Input: part model. Units: mm. Frame: model coordinates. A direction names the side the tool comes from. Give positions to 0.01 mm unless a question says otherwise; leave off trailing zeros. Loops run counter-clockwise (first coordinate to the right, second up) from the corner with the lowest first, then second, coordinate; pieces in that order, holes last. Notation, with made-up numbers: (3.25, 58.5) - (60.25, 58.5) arc R11 ccw to (60.25, 76.5) - close; hole circle Ø2 at (-20.75, 9.5). An arc over 180 degrees is marked (long way). Answer as a JSON object with one key per item and string values. Group by question number.
(1) Section query C-C (z = 16). Return loops of the section in (x, y), plus the area to 3 significant figures.
(2) Material intervals for L1, parallel to Y at x = 0, z = 5.5; L2, parallel to Y at x = -11.5, z = 39; L3, parallel to Z at x = 0, y = -6, sorted ascending.
(3) Section query B-B (y = 0). Return loops of the section in (x, z), plus the area to 3 significant figures.
(4) Section query D-D (y = 7). Return loops of the section in (x, z).
(5) Pin query (flat end, axial travel): P1, Ø1.2, axis at x = 11.5, y = -1, coming from the +Z side; P2, Ø1, axis at x = -5.5, z = 21.5, coming from the +Y side; P3, Ø12, axis at x = 1, z = 38.5, coming from the -Y side. Return the tip coordinate at first contact, or that it passes through.
(6) Section query A-A (x = 0). Return loops of the section in (y, z), plus the area to 3 significant figures.
(7) Mould query, pull axis X, two halves, no side actions, for faces 1 (the cylindrical face through (0, -14, 12)), 2 (the flat face through (14, -5.5, 11)), 3 (the cylindrical face through (-0.91, 6.34, 23.06)), 4 (the cylindrical face through (-9.21, -0.049, 23.985)). Classes: +X half, -X half, draft (parallel to the pull), parting line (faces both ways), or undercut.
(8) Access query for faces 5 (the cylindrical face through (0, 14, 12)), 6 (the flat face through (14, 5.5, 11)), 7 (the cylindrical face through (4.707, -9.049, 9.86)). Directions: +Z, -Z, +X, -X, +Y, -Y. A direction counts if a zero-diameter tool reaches every point of the face in a straight line with its end or side. Return the directions, or none.
```python
from build123d import *

# Parameters (mm, degrees)
CYLINDER002_R          = 11
CYLINDER002_DEPTH      = 7
CYLINDER002_ROLL_ANGLE = -90
BOX_W                  = 30
BOX_H                  = 7
BOX_DEPTH              = 15
BOX001_W               = 10
BOX001_H               = 7
BOX001_DEPTH           = 30
CYLINDER005_R          = 10.2
CYLINDER005_DEPTH      = 20
CYLINDER004_R          = 7
CYLINDER004_DEPTH      = 30
CYLINDER004_ROLL_ANGLE = -90
CYLINDER001_R          = 15
CYLINDER001_DEPTH      = 15
CYLINDER001_ROLL_ANGLE = -90
BOX002_W               = 30
BOX002_H               = 11
BOX002_DEPTH           = 30
CYLINDER_R             = 14
CYLINDER_DEPTH         = 24


with BuildPart() as cylinder002:
    # Cylinder002 → Cylinder002 (new body)
    with BuildSketch(Plane.XY):
        Circle(CYLINDER002_R)
    extrude(amount=CYLINDER002_DEPTH)


with BuildPart() as cylinder002_1:
    # Cylinder002 roll: moved
    add(cylinder002.part.rotate(Axis((0, 0, 0), (1, 0, 0)), CYLINDER002_ROLL_ANGLE))


with BuildPart() as cylinder002_2:
    # Cylinder002 placement: moved
    add(cylinder002_1.part.moved(Location((0, -3.5, 30))))


with BuildPart() as cube:
    # Box → Box (new body)
    with BuildSketch(Plane(origin=(-15, -3.5, 30), x_dir=(1, 0, 0), z_dir=(0, 0, 1))):
        with Locations((15, 3.5)):
            Rectangle(BOX_W, BOX_H)
    extrude(amount=BOX_DEPTH)


with BuildPart() as cube001:
    # Box001 → Box001 (new body)
    with BuildSketch(Plane(origin=(12.5, -3.5, 0), x_dir=(1, 0, 0), z_dir=(0, 0, 1))):
        with Locations((5, 3.5)):
            Rectangle(BOX001_W, BOX001_H)
    extrude(amount=BOX001_DEPTH)


with BuildPart() as cylinder005:
    # Cylinder005 → Cylinder005 (new body)
    with BuildSketch(Plane.XY):
        Circle(CYLINDER005_R)
    extrude(amount=CYLINDER005_DEPTH)


with BuildPart() as obj1:
    # Cylinder004 → Cylinder004 (new body)
    with BuildSketch(Plane.XY):
        Circle(CYLINDER004_R)
    extrude(amount=CYLINDER004_DEPTH)


with BuildPart() as obj1_1:
    # Cylinder004 roll: moved
    add(obj1.part.rotate(Axis((0, 0, 0), (1, 0, 0)), CYLINDER004_ROLL_ANGLE))


with BuildPart() as obj1_2:
    # Cylinder004 placement: moved
    add(obj1_1.part.moved(Location((0, -15, 30))))

    # Fusion001: union Cylinder002, Cube, Cube001, Cylinder005
    add(cylinder002_2.part)
    add(cube.part)
    add(cube001.part)
    add(cylinder005.part)


with BuildPart() as cylinder001:
    # Cylinder001 → Cylinder001 (new body)
    with BuildSketch(Plane.XY):
        Circle(CYLINDER001_R)
    extrude(amount=CYLINDER001_DEPTH)


with BuildPart() as cylinder001_1:
    # Cylinder001 roll: moved
    add(cylinder001.part.rotate(Axis((0, 0, 0), (1, 0, 0)), CYLINDER001_ROLL_ANGLE))


with BuildPart() as cylinder001_2:
    # Cylinder001 placement: moved
    add(cylinder001_1.part.moved(Location((0, -7.5, 30))))


with BuildPart() as cube002:
    # Box002 → Box002 (new body)
    with BuildSketch(Plane(origin=(-15, -5.5, 0), x_dir=(1, 0, 0), z_dir=(0, 0, 1))):
        with Locations((15, 5.5)):
            Rectangle(BOX002_W, BOX002_H)
    extrude(amount=BOX002_DEPTH)


with BuildPart() as cut:
    # Cylinder → Cylinder (new body)
    with BuildSketch(Plane.XY):
        Circle(CYLINDER_R)
    extrude(amount=CYLINDER_DEPTH)

    # Fusion: union Cylinder001, Cube002
    add(cylinder001_2.part)
    add(cube002.part)

    # Cut: cut obj1
    add(obj1_2.part, mode=Mode.SUBTRACT)


solid = cut.part
```
Recorded:
{
 "1": {"outline": "(-15, -5.5) - (-12.87, -5.5) arc R14 ccw to (12.87, -5.5) - (15, -5.5) - (15, -3.5) - (12.5, -3.5) - (12.5, 3.5) - (15, 3.5) - (15, 5.5) - (12.87, 5.5) arc R14 ccw to (-12.87, 5.5) - (-15, 5.5) - close; hole circle Ø20.4 at (0, 0)", "area": "302 mm^2"},
 "2": {"L1": "y = -14 to -10.2, 10.2 to 14", "L2": "y = -7.5 to -3.5, 3.5 to 7.5", "L3": "z = 20 to 23, 37 to 45"},
 "3": {"outline": "(-15, 0) - (-10.2, 0) - (-10.2, 20) - (-4.58, 20) arc R11 cw to (-11, 30) - (-15, 30) - close; (4.58, 20) - (10.2, 20) - (10.2, 0) - (12.5, 0) - (12.5, 30) - (11, 30) arc R11 cw to start", "area": "233 mm^2"},
 "4": {"outline": "(-12.12, 0) - (-7.42, 0) - (-7.42, 20) - (7.42, 20) - (7.42, 0) - (12.12, 0) - (12.12, 21.17) arc R15 ccw (long way) to (-12.12, 21.17) - close; hole circle Ø14 at (0, 30)"},
 "5": {"P1": "stops at z = 30", "P2": "stops at y = 13.08", "P3": "stops at y = -7.5"},
 "6": {"outline": "(-14, 0) - (-10.2, 0) - (-10.2, 20) - (-3.5, 20) - (-3.5, 23) - (-14, 23) - close; (-7.5, 37) - (-3.5, 37) - (-3.5, 45) - (-7.5, 45) - close; (3.5, 20) - (10.2, 20) - (10.2, 0) - (14, 0) - (14, 23) - (3.5, 23) - close; (3.5, 37) - (7.5, 37) - (7.5, 45) - (3.5, 45) - close", "area": "279 mm^2"},
 "7": {"face 1": "parting line", "face 2": "draft", "face 3": "undercut", "face 4": "undercut"},
 "8": {"face 5": "-Z, +Y", "face 6": "-Z, +X, +Y", "face 7": "-Z"}
}
